Autodesk Fusion 360 part; units mm, degrees
sketch "Sketch1" plane through (0, 0, 0) normal (0, 0, 1) x (1, 0, 0)
  line L0 (-40, 20.1) -> (40, 20.1)
  line L1 (40, 20.1) -> (40, -20.1)
  line L2 (40, -20.1) -> (-40, -20.1)
  line L3 (-40, -20.1) -> (-40, 20.1)
  line L4 (-40, 20.1) -> (40, -20.1) construction
  line L5 (40, 20.1) -> (-40, -20.1) construction
  line L6 (0, 20.1) -> (0, 40.1)
  line L7 (0, 40.1) -> (-50, 40.1)
  line L8 (0, -20.1) -> (0, -40.1)
  line L9 (0, -40.1) -> (-50, -40.1)
  line L10 (-40, 0) -> (-70, 0) construction
  circle A0 centre (-70, 0) radius 10.5
  circle A1 centre (-70, 0) radius 30
  line L11 (-80.978, 27.9192) -> (-50, 40.1)
  line L12 (-80.978, -27.9192) -> (-50, -40.1)
  circle A2 centre (-70, 0) radius 4.25
  dimension "d1" = 80
  dimension "d2" = 40.2
  dimension "d3" = 20
  dimension "d4" = 20
  dimension "d5" = 30
  dimension "d6" = 21
  dimension "d7" = 8.5
  dimension "d8" = 10
  dimension "d9" = 10
extrude "Extrude1" add sketch "Sketch1" along normal blind 40 contours L0 L3 L6 L7 A1 L11 | A1 | L2 L3 L8 L9 A1 L12 | A0 makes body 1
sketch "Sketch2" plane through (0, 0, 40) normal (0, 0, 1) x (1, 0, 0)
  circle A0 centre (-70, 0) radius 4.25
  arc A1 (-80.978, 27.9192) -> (-80.978, -27.9192) centre (-70, 0) ccw
  line L0 (-80.978, -27.9192) -> (-50, -40.1)
  line L1 (-50, -40.1) -> (0, -40.1)
  line L2 (0, -40.1) -> (0, -20.1)
  line L3 (0, -20.1) -> (-40, -20.1)
  line L4 (-40, -20.1) -> (-40, 20.1)
  line L5 (-40, 20.1) -> (0, 20.1)
  line L6 (0, 20.1) -> (0, 40.1)
  line L7 (0, 40.1) -> (-50, 40.1)
  line L8 (-50, 40.1) -> (-80.978, 27.9192)
  line L9 (0, 20.1) -> (0, -20.1)
extrude "Extrude2" add sketch "Sketch2" along normal blind 20 bodies 1
sketch "Sketch3" plane through (0, 0, 40) normal (0, 0, -1) x (-1, 0, 0)
  line L0 (40, 20.1) -> (0, 20.1)
  line L1 (0, 20.1) -> (0, -20.1)
  line L2 (0, -20.1) -> (40, -20.1)
  line L3 (40, -20.1) -> (40, 20.1)
  line L4 (20, 20.1) -> (20, -20.1) construction
  circle A0 centre (20, 0) radius 10.5
  circle A1 centre (20, 0) radius 4.25
  dimension "d63" = 21
  dimension "d64" = 8.5
extrude "Extrude16" cut sketch "Sketch3" against normal blind 38 contours A0 | A1 bodies 1
extrude "Extrude17" add sketch "Sketch3" against normal blind 18 contours A0 bodies 1
sketch "Sketch11" plane through (0, 0, 58) normal (0, 0, 1) x (1, 0, 0)
  circle A0 centre (-20, 0) radius 4.25
  circle A1 centre (-20, 0) radius 10.5
  line L0 (-29.6014, 4.25) -> (-10.3986, 4.25)
  line L1 (-10.3986, -4.25) -> (-29.6014, -4.25)
  line L2 (-15.75, 4.25) -> (-15.75, -4.25)
  line L3 (-24.25, 4.25) -> (-24.25, -4.25)
extrude "Extrude18" cut sketch "Sketch11" against normal blind 0.2 contours A0 L1 L2 | A0 L0 L2 | A1 L0 L1 L2 | A0 L0 L3 | A0 L1 L3 | A1 L0 L1 L3 bodies 1
extrude "Extrude19" cut sketch "Sketch11" against normal blind 0.4 contours A0 L1 L2 | A0 L0 L2 | A0 L0 L3 | A0 L1 L3 bodies 1
sketch "Sketch5" plane through (0, 0, 60) normal (0, 0, 1) x (1, 0, 0)
  circle A0 centre (-70, 0) radius 4.25
  line L0 (0, 40.1) -> (-50, 40.1)
  line L1 (-50, 40.1) -> (-80.978, 27.9192)
  arc A1 (-80.978, 27.9192) -> (-80.978, -27.9192) centre (-70, 0) ccw
  line L2 (-80.978, -27.9192) -> (-50, -40.1)
  line L3 (-50, -40.1) -> (0, -40.1)
  line L4 (0, -40.1) -> (0, 40.1)
  circle A2 centre (-70, 0) radius 10.5
  circle A3 centre (-20, 0) radius 10.5
  dimension "d24" = 21
extrude "Extrude5" cut sketch "Sketch5" against normal blind 22 contours A2 bodies 1
sketch "Sketch8" plane through (0, 20.1, 0) normal (0, -1, 0) x (1, 0, 0)
  line L0 (-40, 0) -> (0, 0)
  line L1 (0, 0) -> (0, 40)
  line L2 (0, 40) -> (-40, 40)
  line L3 (-40, 40) -> (-40, 0)
  line L4 (-40, 40) -> (0, 0) construction
  circle A0 centre (-20, 20) radius 4.25
  circle A1 centre (-20, 20) radius 10.5
  dimension "d42" = 8.5
  dimension "d43" = 21
extrude "Extrude9" cut sketch "Sketch8" along normal blind -43 and the other way blind -83 contours A0 | A1 bodies 1
extrude "Extrude10" add sketch "Sketch8" against normal blind 18 contours A1 bodies 1
extrude "Extrude11" add sketch "Sketch8" along normal blind 18 from surface at 40.2 contours A1 bodies 1
sketch "Sketch10" plane through (0, 0, 38) normal (0, 0, 1) x (1, 0, 0)
  circle A0 centre (-70, 0) radius 4.25
  circle A1 centre (-70, 0) radius 10.5
  line L0 (-74.25, 9.6014) -> (-74.25, -9.6014)
  line L1 (-65.75, 9.6014) -> (-65.75, -9.6014)
  line L2 (-74.25, 4.25) -> (-65.75, 4.25)
  line L3 (-65.75, -4.25) -> (-74.25, -4.25)
extrude "Extrude14" cut sketch "Sketch10" against normal blind 0.2 contours A0 L1 L3 | A0 L1 L2 | A0 L0 L2 | A1 L0 L1 L2 | A0 L0 L3 | A1 L0 L1 L3 bodies 1
extrude "Extrude15" cut sketch "Sketch10" against normal blind 0.4 contours A0 L1 L3 | A0 L1 L2 | A0 L0 L2 | A0 L0 L3 bodies 1
extrude "Extrude20" add 1 faces at (-48.5833, 0, 0) along direction (0, 0, -1) blind 10 on bodies 1 bodies 1
sketch "Sketch12" plane through (-40, 0, 0) normal (1, 0, 0) x (0, 0, -1)
  line L0 (10, 20.1) -> (-40, 20.1)
  line L1 (-40, 20.1) -> (-40, -20.1)
  line L2 (-40, -20.1) -> (10, -20.1)
  line L3 (10, -20.1) -> (10, 20.1)
  line L4 (1, 20.1) -> (1, -20.1)
  dimension "d85" = 41
extrude "Extrude21" add sketch "Sketch12" along normal blind 40 contours L0 L2 L3 L4 bodies 1
fillet "Fillet2" radius 80 2 edges at (-50, 40.1, 30) (-50, -40.1, 30) on bodies 1
fillet "Fillet2" radius 7.5 2 edges at (0, 40.1, 30) (0, -40.1, 30) on bodies 1
chamfer "Chamfer1" distance 4 distance2 4 10 edges at (-49.7348, 38.7006, 60) (-21.1684, 40.1, 60) (-2.1967, 37.9033, 60) (0, 0, 60) (-2.1967, -37.9033, 60) (-21.1684, -40.1, 60) (-49.7348, -38.7006, 60) (-72.5448, -31.2352, 60) (-100, 0, 60) (-72.5448, 31.2352, 60) measured on face at (-51.3673, 38.3735, 36.6667) measured on face at (-44.9337, 17.1022, 60) measured on face at (-7.1431, 40.0915, 36.6667) measured on face at (-44.9337, 17.1022, 60) measured on face at (-7.1431, -40.0915, 13.3333) measured on face at (-44.9337, 17.1022, 60) measured on face at (-38.1659, -40.0307, 13.3333) measured on face at (-44.9337, 17.1022, 60) measured on face at (-44.9337, 17.1022, 60) measured on face at (-44.9337, 17.1022, 60) on bodies 1
chamfer "Chamfer1" distance 0.4 distance2 0.4 2 edges at (-16.0376, 1.5369, 40) (-73.9624, -1.5369, -10) 2 faces at (-15.7553, -32.1, 19.7882) (-15.7553, 32.1, 19.7882) measured on face at (-20.1059, -14.8127, 40) measured on face at (-21.9167, 0, -10) on bodies 1
fillet "Fillet3" radius 1 2 edges at (0, -20.1, 20) (0, 20.1, 20) on bodies 1
copy_body "Body->Comp1" bodies 1 removing the originals makes body 2 in component "side brace upper mount"
component "side brace upper mount" placed x (1, 0, 0) y (0, 1, 0) z (0, 0, 1) at (0, 0, 0)
Read the model definition and answer for the solid it produces. Units are mm, in the model's axes. A direction names the side the tool comes from. Coordinates: 2 decimals unless noted, no trailing zeros. Order: outer loops, then holes, each group sorted by start corner. A loop starts at its lowest first (then second) coordinate and runs counter-clockwise, first axis right, second up. Notation, with made-up numbers: (31, -0.5) - (57, -0.5) arc R14 cw to (57, 9.5) - close; hole circle Ø7 at (6.25, 50.25). An arc over 180 degrees is marked (long way). Answer as a JSON object with one key per item and string values. Group by question number.
Item 1: Section C-C (x = -77) is taken. Give the vertices of the cut face in (y, z), plus the area to 3 significant figures.
Item 2: Flat-ended cylindrical pins translate along their axes: P1, Ø12, axis at x = -66, z = 5.5, coming from the -Y side; P2, Ø2, axis at x = -23, y = 3, coming from the +Z side; P3, Ø1.9, axis at x = -62.5, y = 4, coming from the +Z side. Find the tip coordinate at first contact, or state that the pin passes through.
Item 3: Section A-A (z = 43) is taken. Give the vertices of the cut face in (x, y).
Item 4: Consider probe 1 along X at (y, z) = (0, 53.5); probe 2 along Z at (x, y) = (-4.5, -5); probe 3 along Z at (x, y) = (-20, -30). Determine where each line is inside the solid, lowest interval first. Write a range as from..to.
Item 5: Section D-D (z = 33) is taken. Give the vertices of the cut face in (x, y), plus the area to 3 significant figures.
Item 6: A tool of negligible diameter and unlimited length cuts with its end or side. For faces 4 (the face through (-70, -7, 37.8)), 5 (the face through (-71.92, 29.3, 58.03)), from which of +Z, -Z, +X, -X, +Y, -Y can it reach the whole face along a straight path? Write none if from no direction.
Item 7: The mould has two halves that part along Z. Classify faces 1 (the face through (-21, -38.1, 58)), 2 (the face through (-40, 0, 20)), 3 (the face through (-99.996, -0.502, 47.888)): +Z half, -Z half, draft (parallel to the pull), parting line (faces both ways), or undercut.
Item 8: Section B-B (y = 29.5) is taken. Give the vertices of the cut face in (x, z).
Results are:
{
 "1": {"outline": "(-29.48, -10) - (29.48, -10) - (29.48, 56) - (25.19, 60) - (7.83, 60) - (7.83, 38) - (-7.83, 38) - (-7.83, 60) - (-25.19, 60) - (-29.48, 56) - close", "area": "3,770 mm^2"},
 "2": {"P1": "stops at y = -36.04", "P2": "stops at z = 57.6", "P3": "stops at z = 38"},
 "3": {"outline": "(-80.98, -27.92) - (-64.11, -34.55) arc R80 ccw to (-34.84, -40.1) - (-7.5, -40.1) arc R7.5 ccw to (0, -32.6) - (0, 32.6) arc R7.5 ccw to (-7.5, 40.1) - (-34.84, 40.1) arc R80 ccw to (-64.11, 34.55) - (-80.98, 27.92) arc R30 ccw to start; hole circle Ø21 at (-70, 0); hole circle Ø8.5 at (-20, 0)"},
 "4": {"probe 1": "x = -100..-80.5, -59.5..-24.25, -15.75..0", "probe 2": "z = -10..-1, 40..60", "probe 3": "z = -10..15.75, 24.25..60"},
 "5": {"outline": "(-80.98, -27.92) - (-64.11, -34.55) arc R80 ccw to (-34.84, -40.1) - (-7.5, -40.1) arc R7.5 ccw to (0, -32.6) - (0, -21.1) arc R1 ccw to (-1, -20.1) - (-40, -20.1) - (-40, 20.1) - (-1, 20.1) arc R1 ccw to (0, 21.1) - (0, 32.6) arc R7.5 ccw to (-7.5, 40.1) - (-34.84, 40.1) arc R80 ccw to (-64.11, 34.55) - (-80.98, 27.92) arc R30 ccw to start; hole circle Ø8.5 at (-70, 0)", "area": "5,170 mm^2"},
 "6": {"face 4": "+Z", "face 5": "+Z, -X, +Y"},
 "7": {"face 1": "+Z half", "face 2": "undercut", "face 3": "draft"},
 "8": {"outline": "(-76.96, -10) - (0, -10) - (0, 56) - (-4, 60) - (-66.03, 60) - (-76.96, 56) - close; hole circle Ø8.5 at (-20, 20)"}
}
